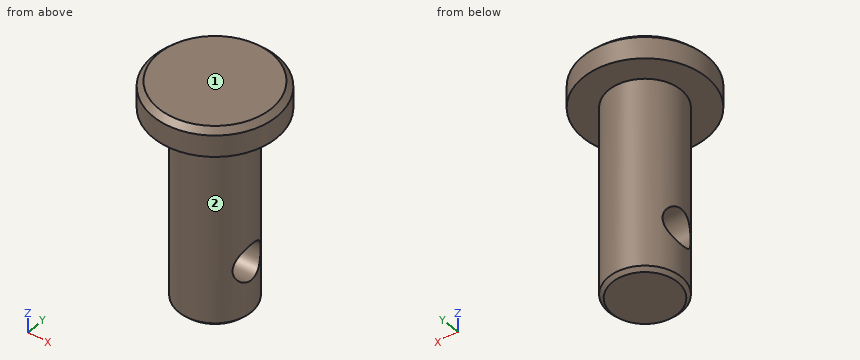
from build123d import *

# Parameters (mm, degrees)
SKETCH1_R           = 2.38125
EXTRUDE1_DEPTH      = 6.35
SKETCH2_R           = 4.064
EXTRUDE2_DEPTH      = 1.778
CHAMFER1_SIZE       = 0.3556
SKETCH3_R           = 1.190625
EXTRUDE3_DEPTH      = 5.064
EXTRUDE3_DEPTH_BACK = 5.064
CHAMFER2_SIZE       = 0.238125


with BuildPart() as part:
    # Sketch1 → Extrude1 (new body, symmetric)
    with BuildSketch(Plane.XY):
        Circle(SKETCH1_R)
    extrude(amount=EXTRUDE1_DEPTH, both=True)

    # Sketch2 → Extrude2 (add)
    with BuildSketch(Plane.XY.offset(6.35)):
        Circle(SKETCH2_R)
    extrude(amount=EXTRUDE2_DEPTH)

    # Chamfer1
    chamfer1_edges = [part.edges().sort_by_distance(p)[0] for p in [
        (-4.064, 0, 8.128),
    ]]
    chamfer(chamfer1_edges, length=CHAMFER1_SIZE)

    # Sketch3 → Extrude3 (cut, two sides)
    with BuildSketch(Plane(origin=(0, 0, 0), x_dir=(0, 0, -1), z_dir=(1, 0, 0))) as extrude3_sk:
        with Locations((2.778125, 0)):
            Circle(SKETCH3_R)
    extrude(amount=EXTRUDE3_DEPTH, mode=Mode.SUBTRACT)
    extrude(extrude3_sk.sketch, amount=-EXTRUDE3_DEPTH_BACK, mode=Mode.SUBTRACT)

    # Chamfer2
    chamfer2_edges = [part.edges().sort_by_distance(p)[0] for p in [
        (-2.38125, 0, -6.35),
    ]]
    chamfer(chamfer2_edges, length=CHAMFER2_SIZE)


solid = part.part
The listing builds one solid part. Answer for the finished solid, in the listing's coordinates (mm). Face numbers are marked on the shaded views. A direction names the side the tool comes from. Coordinates: 2 decimals unless noted, no trailing zeros. Order: outer loops, then holes, each group sorted by start corner. A loop starts at its lowest first (then second) coordinate and runs counter-clockwise, first axis right, second up. Notation, with made-up numbers: (68.25, -20.75) -> (79.25, -20.75) arc R27 cw to (79.25, -4.75) -> close; hole circle Ø11 at (-33, 1.5). An arc over 180 degrees is marked (long way). Answer in a Markdown table with one row per item. Add a question column.
Item 1: Find the intervals of material crossed by L1, parallel to Z at x = -1.1, y = 0; L2, parallel to Z at x = -1.25, y = -3.25; L3, parallel to X at y = 0, z = 4, in increasing order. Write a range as from..to.
Item 2: Find section A-A (y = 0). Write down the section's boundary in (x, z).
Item 3: Each of these flat-tipped pins is pushed along its axis until it touches: P1, Ø1, axis at x = 0, z = 0, coming from the +Y side; P2, Ø1.9, axis at y = 0, z = -2.78, coming from the +X side; P3, Ø4, axis at y = 0, z = -2.78, coming from the +X side. Where does it stop, or does it pass through?
Item 4: Which of the six approach directions +Z, -Z, +X, -X, +Y, -Y give full straight-line access (tool end or side, diameter ignored) to the marked faces 1 and 2?
Item 5: Find section B-B (z = 6.75). Write down the section's boundary in (x, y), then the cut area to 3 significant figures.
Result set:
| question | item | result |
|---|---|---|
| 1 | L1 | z = -6.35..-3.97, -1.59..8.13 |
| 1 | L2 | z = 6.35..8.13 |
| 1 | L3 | x = -2.38..2.38 |
| 2 | outline | (-4.06, 6.35) -> (-2.38, 6.35) -> (-2.38, -1.59) -> (2.38, -1.59) -> (2.38, 6.35) -> (4.06, 6.35) -> (4.06, 7.77) -> (3.71, 8.13) -> (-3.71, 8.13) -> (-4.06, 7.77) -> close; (-2.38, -6.11) -> (-2.14, -6.35) -> (2.14, -6.35) -> (2.38, -6.11) -> (2.38, -3.97) -> (-2.38, -3.97) -> close |
| 3 | P1 | stops at y = 2.38 |
| 3 | P2 | passes through |
| 3 | P3 | stops at x = 2.38 |
| 4 | face 1 | +Z, +X, -X, +Y, -Y |
| 4 | face 2 | -Z |
| 5 | outline | circle Ø8.13 at (0, 0) |
| 5 | area | 51.9 mm² |
